Print and shaded views of the part. All mm, measured from the part's lowest x, y and z. Coordinates: 2 decimals unless noted, no trailing zeros. Order: outer loops, then holes, each group sorted by start corner. A loop starts at its lowest first (then second) coordinate and runs counter-clockwise, first axis right, second up. Notation, with made-up numbers: (60.25, -8) -> (78.25, -8) arc R13 cw to (78.25, 17) -> close; hole circle Ø4 at (-31.75, 9). An arc over 180 degrees is marked (long way). Use one line per item in the form item = value. Start each with the question number.
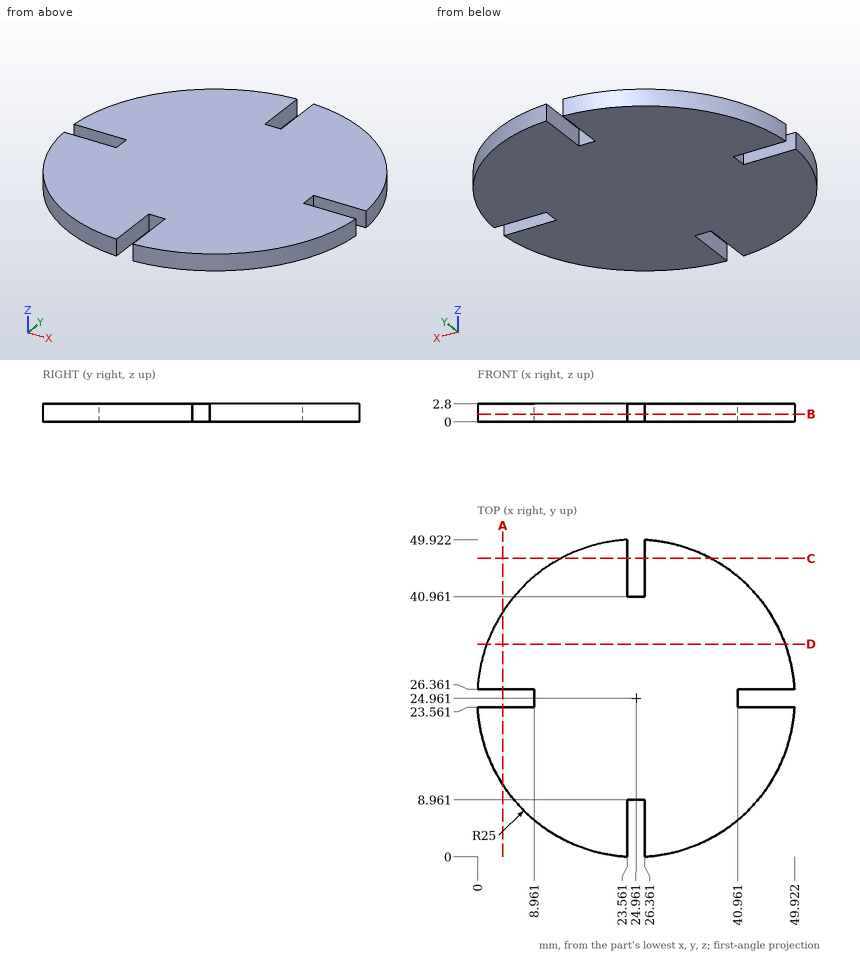
1) Cut at C-C on y = 47. Give the cut face in (x, z).
2) Probe L1, parallel to X at y = 8.5, z = 2.2 (1 decimal); L2, parallel to X at y = 6.5, z = 1.3 (1 decimal); L3, parallel to Y at x = 5.5, z = 2.7 (1 decimal). List the from-to ranges inside material, lowest first.
3) Cut at A-A on x = 4. Give the cut face in (y, z) (1 decimal).
4) Drop flat-ended pins along their axis: P1, Ø1.4, axis at x = 2.5, z = 1.5, coming from the -Y side (1 decimal); P2, Ø1.4, axis at y = 45.5, z = 1.5, coming from the -X side; P3, Ø0.8, axis at x = 43.5, z = 1.5, coming from the -Y side; P4, Ø2, axis at x = 22, y = 13.5, coming from the -Z side. Give the stop position or say it passes through.
5) Cut at D-D on y = 33.5. Give the cut face in (x, z) (1 decimal).
6) Cut at B-B on z = 1.2. Give the cut face in (x, y).
Values follow:
q1.outline = (13.16, 0) -> (23.56, 0) -> (23.56, 2.8) -> (13.16, 2.8) -> close; (26.36, 0) -> (36.76, 0) -> (36.76, 2.8) -> (26.36, 2.8) -> close
q2.L1 = 6.1 to 23.6, 26.4 to 43.8
q2.L2 = 8.1 to 23.6, 26.4 to 41.8
q2.L3 = 9.3 to 23.6, 26.4 to 40.7
q3.outline = (11.3, 0) -> (23.6, 0) -> (23.6, 2.8) -> (11.3, 2.8) -> close; (26.4, 0) -> (38.6, 0) -> (38.6, 2.8) -> (26.4, 2.8) -> close
q4.P1 = 12.7
q4.P2 = 9.75
q4.P3 = 7.76
q4.P4 = 0
q5.outline = (1.5, 0) -> (48.5, 0) -> (48.5, 2.8) -> (1.5, 2.8) -> close
q6.outline = (0, 23.56) arc R25 ccw to (23.56, 0) -> (23.56, 8.96) -> (26.36, 8.96) -> (26.36, 0) arc R25 ccw to (49.92, 23.56) -> (40.96, 23.56) -> (40.96, 26.36) -> (49.92, 26.36) arc R25 ccw to (26.36, 49.92) -> (26.36, 40.96) -> (23.56, 40.96) -> (23.56, 49.92) arc R25 ccw to (0, 26.36) -> (8.96, 26.36) -> (8.96, 23.56) -> close
